from build123d import *
from build123d import SkipClean  # not in build123d's __all__

# Parameters (mm, degrees)
F2_R     = 8
F2_R_2   = 42.5
F0_DEPTH = 25


with BuildPart() as f0:
    # F2 (on Top) → F0 (new body)
    with BuildSketch(Plane.XY):
        with BuildLine():
            Line((0, -12), (0, 0))
            Line((0, 0), (-240, 0))
            ThreePointArc((-240, 0), (-247.0710678119, -2.9289321881), (-250, -10))
            Line((-250, -10), (-250, -140))
            ThreePointArc((-250, -140), (-247.0710678119, -147.0710678119), (-240, -150))
            Line((-240, -150), (0, -150))
            Line((0, -150), (0, -138))
            ThreePointArc((0, -138), (-8, -130), (0, -122))
            Line((0, -122), (0, -28))
            ThreePointArc((0, -28), (-8, -20), (0, -12))
        make_face()
        with Locations((-230, -130)):
            Circle(F2_R, mode=Mode.SUBTRACT)
        with Locations((-115, -130)):
            Circle(F2_R, mode=Mode.SUBTRACT)
        with Locations((-172.5, -75)):
            Circle(F2_R_2, mode=Mode.SUBTRACT)
        with Locations((-230, -20)):
            Circle(F2_R, mode=Mode.SUBTRACT)
        with Locations((-57.5, -75)):
            Circle(F2_R_2, mode=Mode.SUBTRACT)
        with Locations((-115, -20)):
            Circle(F2_R, mode=Mode.SUBTRACT)
    extrude(amount=F0_DEPTH)

    # F1: F0 across face


with BuildPart() as f0_1:
    add(f0.part, clean=False)
    with SkipClean():  # cleaning this boolean's faces spoils the solid; the shape is the same uncleaned
        add(f0.part.mirror(Plane(origin=(0, -75, 12.5), x_dir=(0, 1, 0), z_dir=(1, 0, 0))), clean=False)


solid = f0_1.part
Design review of the part built by this model. Coordinates are the model's own, in mm. Round coordinates to 2 decimals unless told otherwise and drop trailing zeros. Order: outer loops, then holes, each group sorted by start corner. A loop starts at its lowest first (then second) coordinate and runs counter-clockwise, first axis right, second up. Notation, with made-up numbers: M 27,-24.5 L 32,-24.5 A9 ccw 32,-12.5 Z; hole C -9,-3 d2. An arc over 180 degrees is marked long. Answer as CSV lines item,"result". Start each with the question number.
1) For pin 1 Ø13 at (x, y) = (0, -130) entering from -Z, flat-tipped, find the tip position at first contact; note if it passes through.
2) Add section A-A (z = 7.5). Give the number of separate pieces and of enclosed holes in the cut face, then the cut area to 3 significant figures.
3) Add section D-D (y = -20). Give the boundary of the cut face in (x, z).
4) The part is to be moulded in two halves that separate along X. For faces 1 (the face through (3, -74, 0)), 2 (the face through (226.31, -137.1, 12.32)), 3 (the face through (-246.99, -2.85, 12.32)), say which applies: +X half, -X half, draft (parallel to the pull), parting line (faces both ways), or undercut.
5) Add section B-B (y = -41). Give the boundary of the cut face in (x, z), then the cut area to 3 significant figures.
6) Add section C-C (x = -115). Give the boundary of the cut face in (y, z), then the cut area to 3 significant figures.
7) Wall thickness on line 1 along Y through (x, z) = (230, 8); line 2 along X through (y, z) = (-130.5, 15); line 3 along Y through (x, z) = (172.5, 10.5): over which ranges is each line inside the solid? List them lowest first. Write a range as [from, to].
Resolved:
1,pin 1,"through"
2,separate pieces,"1"
2,enclosed holes,"14"
2,area,"50,200 mm^2"
3,outline,"M -250,0 L -238,0 L -238,25 L -250,25 Z; M -222,0 L -123,0 L -123,25 L -222,25 Z; M -107,0 L -8,0 L -8,25 L -107,25 Z; M 8,0 L 107,0 L 107,25 L 8,25 Z; M 123,0 L 222,0 L 222,25 L 123,25 Z; M 238,0 L 250,0 L 250,25 L 238,25 Z"
4,face 1,"draft"
4,face 2,"undercut"
4,face 3,"-X half"
5,outline,"M -250,0 L -198,0 L -198,25 L -250,25 Z; M -147,0 L -83,0 L -83,25 L -147,25 Z; M -32,0 L 32,0 L 32,25 L -32,25 Z; M 83,0 L 147,0 L 147,25 L 83,25 Z; M 198,0 L 250,0 L 250,25 L 198,25 Z"
5,area,"7,400 mm^2"
6,outline,"M -150,0 L -138,0 L -138,25 L -150,25 Z; M -122,0 L -28,0 L -28,25 L -122,25 Z; M -12,0 L 0,0 L 0,25 L -12,25 Z"
6,area,"2,950 mm^2"
7,line 1,"[-150, -138], [-122, -28], [-12, 0]"
7,line 2,"[-250, -237.98], [-222.02, -122.98], [-107.02, -7.98], [7.98, 107.02], [122.98, 222.02], [237.98, 250]"
7,line 3,"[-150, -117.5], [-32.5, 0]"
